Input: part model. Units: mm. Frame: model coordinates. A direction names the side the tool comes from. Round coordinates to 2 decimals unless told otherwise and drop trailing zeros. Write each loop counter-clockwise with the first axis right and the second up, starting at its lowest first coordinate (ties: lowest second). Pieces come first, ordered by that corner, then holes. Notation, with made-up numbers: (30.5, 57.5) -> (43.5, 57.5) arc R30 ccw to (43.5, 82.5) -> close; hole circle Ø1 at (-9, 54). An arc over 180 degrees is marked (long way). Use CSV: the item, a comma, the result in double quotes.
```python
from build123d import *

# Parameters (mm, degrees)
F0_W          = 2.528925892
F0_H          = 2.5279636029
F1_DEPTH      = 56.0451
F1_DEPTH_BACK = 56.0451
F2_R          = 2.1639792623
F3_DEPTH      = 2.286


# Not quite as in the source:
# - a pattern or mirror of a feature is missing from the dataset's text; its kind, count and spacing are read off the source's solid


with BuildPart() as f1:
    # F0 (on Front) → F1 (new body, two sides)
    with BuildSketch(Plane.XZ) as f1_sk:
        Rectangle(F0_W, F0_H)
    extrude(amount=F1_DEPTH)
    extrude(f1_sk.sketch, amount=-F1_DEPTH_BACK)

    # F2 (on face) → F3 (join)
    with BuildSketch(Plane.XZ.offset(56.0451)):
        Circle(F2_R)
    f3 = extrude(amount=F3_DEPTH)

    # F3_copies: F3 across plane
    add(f3.mirror(Plane.ZX))


solid = f1.part
```
Item 1: Set-up query: faces 5 (the face through (1.264, -1, 0)), 6 (the face through (0, 58.331, 0)), 7 (the face through (-1.264, -1, 0)). Return all of +Z, -Z, +X, -X, +Y, -Y with unobstructed straight access to the full face (end or side cutting, diameter ignored); none if empty.
Worked answers:
face 5,"+Z, -Z, +X"
face 6,"+Z, -Z, +X, -X, +Y"
face 7,"+Z, -Z, -X"
Item 2: Pull-direction query (Y, two-part tool) for faces 1 (the face through (0, -1, 1.264)), 2 (the face through (-0.469, 57.172, -2.113)), 3 (the face through (0, -1, -1.264)), 4 (the face through (0, -58.331, 0)); classes: +Y half, -Y half, draft (parallel to the pull), parting line (faces both ways), or undercut.
Worked answers:
face 1,"undercut"
face 2,"draft"
face 3,"undercut"
face 4,"-Y half"
Item 3: Section query B-B on x = 0. Return the cut outline in (y, z), plus the area to 3 significant figures.
Worked answers:
outline,"(-58.33, -2.16) -> (-56.05, -2.16) -> (-56.05, -1.26) -> (56.05, -1.26) -> (56.05, -2.16) -> (58.33, -2.16) -> (58.33, 2.16) -> (56.05, 2.16) -> (56.05, 1.26) -> (-56.05, 1.26) -> (-56.05, 2.16) -> (-58.33, 2.16) -> close"
area,"303 mm²"
Item 4: Section query C-C on y = 19.5. Return the cut outline in (x, z), plus the area to 3 significant figures.
Worked answers:
outline,"(-1.26, -1.26) -> (1.26, -1.26) -> (1.26, 1.26) -> (-1.26, 1.26) -> close"
area,"6.39 mm²"
Item 5: Section query A-A on z = 0. Return the cut outline in (x, y), plus the area to 3 significant figures.
Worked answers:
outline,"(-2.16, -58.33) -> (2.16, -58.33) -> (2.16, -56.05) -> (1.26, -56.05) -> (1.26, 56.05) -> (2.16, 56.05) -> (2.16, 58.33) -> (-2.16, 58.33) -> (-2.16, 56.05) -> (-1.26, 56.05) -> (-1.26, -56.05) -> (-2.16, -56.05) -> close"
area,"303 mm²"
Item 6: First-contact query: pin 1 Ø1.3 at (y, z) = (-9.5, -0.5) entering from -X; pin 2 Ø2 at (y, z) = (3, 0) entering from +X; pin 3 Ø1.3 at (x, y) = (0, 18) entering from +Z. Flat tips, straight axial feed; report the tip coordinate or a pass-through.
Worked answers:
pin 1,"stops at x = -1.26"
pin 2,"stops at x = 1.26"
pin 3,"stops at z = 1.26"
Item 7: Line query: line 1 (Y direction, x = -1.3, z = 1.2); line 2 (Z direction, x = 0.85, y = 0). Output: solid intervals per line, ascending.
Worked answers:
line 1,"y = -58.33 to -56.05, 56.05 to 58.33"
line 2,"z = -1.26 to 1.26"
